Part model, mm, in its own coordinate system. A direction names the side the tool comes from. Coordinates: 2 decimals unless noted, no trailing zeros. Write each loop counter-clockwise with the first axis right and the second up, starting at its lowest first coordinate (ties: lowest second). Pieces come first, ordered by that corner, then holes. Notation, with made-up numbers: (52, 66.25) -> (84, 66.25) arc R7 ccw to (84, 79.25) -> close; hole circle Ø6 at (1.25, 2.25). An arc over 180 degrees is marked (long way). Write item = value, one per line. Start each with the question number.
Q1. Probe line 1 (Y direction, x = -30, z = -110); line 2 (Z direction, x = -20.5, y = 10.75); line 3 (X direction, y = -6.5, z = -54). List the from-to ranges inside material, lowest first.
Q2. Band-saw the part on C-C, the plane z = -60.5. List the corners of the cut face in (x, y).
Q3. Tool access for faces 4 (the cylindrical face through (-25, 0, -110)), 5 (the flat face through (-24, 0, -107.5)), 6 (the flat face through (-50.98, 2.78, -15)), 7 (the cylindrical face through (-0.35, 0.17, -0.51)), 8 (the flat face through (-50, 0, -110)): list every direction of +Z, -Z, +X, -X, +Y, -Y with a clear straight run to the whole face (end or side of a thin tool).
Q4. Band-saw the part on A-A, the plane x = -23.5. List the corners of the cut face in (y, z), plus the area to 3 significant figures.
Q5. Pin check, flat tips, straight feed: P1, Ø1, axis at y = -6.5, z = -38, coming from the -X side; P2, Ø5.5, axis at y = -4.5, z = -110.5, coming from the -X side; P3, Ø12, axis at x = -51, y = 5.5, coming from the +Z side. Stop position of each tip, or through.
Q6. Pull direction Z, two halves, no side cores. Call faces 1 (the flat face through (2.5, 0, -54)), 2 (the flat face through (-73.3, 0.2, -25)), 3 (the flat face through (-18, 0, -2.5)): released by +Z, released by -Z, zero draft, split by the parting line, or undercut.
Q7. Band-saw the part on B-B, the plane y = -3.75. List the corners of the cut face in (x, z), plus the area to 3 significant figures.
from build123d import *

# Parameters (mm, degrees)
EXTRUDE_THIN1_DEPTH = 11.787987944
FILLET1_R           = 5
FILLET2_R           = 10
FILLET3_R           = 10
FILLET4_R           = 5
FILLET5_R           = 5
FILLET6_R           = 10
SKETCH3_R           = 5
CUT_EXTRUDE1_DEPTH  = 10
SKETCH5_R           = 5
CUT_EXTRUDE2_DEPTH  = 10


with BuildPart() as part:
    # Sketch1 → Extrude-Thin1 (new, symmetric)
    with BuildSketch(Plane(origin=(0, 0, 0), x_dir=(1, 0, 0), z_dir=(0, 1, 0))):
        Polygon((-50, 107.5), (-2.5, 107.5), (-2.5, 2.5), (-29.330127019, 2.5), (-72.051270189, 27.165063509), (-74.551270189, 22.834936491), (-30.669872981, -2.5), (2.5, -2.5), (2.5, 112.5), (-50, 112.5), align=None)
    extrude(amount=EXTRUDE_THIN1_DEPTH, both=True)

    # Fillet1
    fillet1_edges = [part.edges().sort_by_distance(p)[0] for p in [
        (-2.5, 0, -107.5),
    ]]
    fillet(fillet1_edges, radius=FILLET1_R)

    # Fillet2
    fillet2_edges = [part.edges().sort_by_distance(p)[0] for p in [
        (2.5, 0, -112.5),
    ]]
    fillet(fillet2_edges, radius=FILLET2_R)

    # Fillet3
    fillet3_edges = [part.edges().sort_by_distance(p)[0] for p in [
        (2.5, 0, 2.5),
    ]]
    fillet(fillet3_edges, radius=FILLET3_R)

    # Fillet4
    fillet4_edges = [part.edges().sort_by_distance(p)[0] for p in [
        (-2.5, 0, -2.5),
    ]]
    fillet(fillet4_edges, radius=FILLET4_R)

    # Fillet5
    fillet5_edges = [part.edges().sort_by_distance(p)[0] for p in [
        (-29.330127019, 0, -2.5),
    ]]
    fillet(fillet5_edges, radius=FILLET5_R)

    # Fillet6
    fillet6_edges = [part.edges().sort_by_distance(p)[0] for p in [
        (-30.669872981, 0, 2.5),
    ]]
    fillet(fillet6_edges, radius=FILLET6_R)

    # Sketch3 → Cut-Extrude1 (cut)
    with BuildSketch(Plane(origin=(0, 0, -112.5), x_dir=(-1, 0, 0), z_dir=(0, 0, -1))):
        with Locations((30, 0)):
            Circle(SKETCH3_R)
    extrude(amount=-CUT_EXTRUDE1_DEPTH, mode=Mode.SUBTRACT)

    # Sketch5 → Cut-Extrude2 (cut)
    with BuildSketch(Plane(origin=(-8.75, 0, 15.155444566), x_dir=(0.866025403784438, 0, 0.500000000000001), z_dir=(-0.500000000000001, 0, 0.866025403784438))):
        with Locations((-55.980762114, -1.07656789)):
            Circle(SKETCH5_R)
    extrude(amount=-CUT_EXTRUDE2_DEPTH, mode=Mode.SUBTRACT)


solid = part.part
Ans:
q1.line_1 = -11.79 to -5, 5 to 11.79
q1.line_2 = -112.5 to -107.5, -2.5 to 2.5
q1.line_3 = -2.5 to 2.5
q2.outline = (-2.5, -11.79) -> (2.5, -11.79) -> (2.5, 11.79) -> (-2.5, 11.79) -> close
q3.face_4 = -Z
q3.face_5 = -X, +Y, -Y
q3.face_6 = +Y, -Y
q3.face_7 = +Z, +X, +Y, -Y
q3.face_8 = -Z, -X, +Y, -Y
q4.outline = (-11.79, -112.5) -> (11.79, -112.5) -> (11.79, -107.5) -> (-11.79, -107.5) -> close; (-11.79, -2.5) -> (11.79, -2.5) -> (11.79, 2.5) -> (-11.79, 2.5) -> close
q4.area = 236 mm2
q5.P1 = -2.5
q5.P2 = -50
q5.P3 = -5.77
q6.face_1 = zero draft
q6.face_2 = released by -Z
q6.face_3 = undercut
q7.outline = (-74.55, -22.83) -> (-72.05, -27.17) -> (-58.39, -19.28) -> (-60.89, -14.95) -> close; (-53.57, -10.72) -> (-51.07, -15.05) -> (-30.49, -3.17) arc R5 cw to (-27.99, -2.5) -> (-7.5, -2.5) arc R5 cw to (-2.5, -7.5) -> (-2.5, -102.5) arc R5 cw to (-7.5, -107.5) -> (-26.69, -107.5) -> (-26.69, -112.5) -> (-7.5, -112.5) arc R10 ccw to (2.5, -102.5) -> (2.5, -7.5) arc R10 ccw to (-7.5, 2.5) -> (-27.99, 2.5) arc R10 ccw to (-32.99, 1.16) -> close; (-50, -112.5) -> (-33.31, -112.5) -> (-33.31, -107.5) -> (-50, -107.5) -> close
q7.area = 1,090 mm2
